Model file for the job. Use its own axes, mm. Round coordinates to 2 decimals unless told otherwise and drop trailing zeros. Loops run counter-clockwise (first coordinate to the right, second up) from the corner with the lowest first, then second, coordinate; pieces in that order, holes last. Notation, with made-up numbers: M 21.5,55.5 L 62.5,55.5 A24 ccw 62.5,71.5 Z; hole C 10.25,8.25 d8. An arc over 180 degrees is marked long. Use a Markdown table: item, result. Add a question column.
Item 1: Pin check, flat tips, straight feed: P1, Ø2, axis at x = 1, y = 12.5, coming from the -Z side; P2, Ø1.8, axis at y = 1.5, z = -2, coming from the -X side; P3, Ø2, axis at x = 0.5, y = 15.5, coming from the +Z side. Stop position of each tip, or through.
Item 2: Saw through at C-C on x = 493. Write the cut outline in (y, z).
Item 3: Saw through at B-B on y = 9. Write the cut outline in (x, z), then the cut area to 3 significant figures.
Item 4: Wall check: L1, parallel to Y at x = 603, z = -174; L2, parallel to Z at x = 384, y = 22.5; L3, parallel to Z at x = 288, y = 27.5. Give the ranges that are in metal, low to high. Write a range as from..to.
Item 5: Saw through at A-A on z = -30. Write the cut outline in (x, y).
Item 6: Two-plate mould, pull along Z, no slides. Class faces 1 (the flat face through (700, 15, -222)), 2 (the flat face through (345, 15, 0)), 3 (the flat face through (345, 2, -222)): +Z half, -Z half, draft (parallel to the pull), parting line (faces both ways), or undercut.
```python
from build123d import *

# Parameters (mm, degrees)
SKETCH2_W                  = 700
SKETCH2_H                  = 450
BOSS_EXTRUDE1_DEPTH        = 30
CONVERT_SOLID1_START       = 3
CONVERT_SOLID1_DEPTH       = 694
CONVERT_SOLID1_2_OUTLINE_W = 24.146446609
CONVERT_SOLID1_2_OUTLINE_H = 2
CONVERT_SOLID1_2_DEPTH     = 2.353553391
CONVERT_SOLID1_START_2     = 697.646446609
CONVERT_SOLID1_3_OUTLINE_W = 24.146446609
CONVERT_SOLID1_3_OUTLINE_H = 2
CONVERT_SOLID1_3_DEPTH     = 2.353553391
CONVERT_SOLID1_4_DEPTH     = 700
CONVERT_SOLID1_5_DEPTH     = 2.353553391
CONVERT_SOLID1_6_DEPTH     = 2.353553391
CONVERT_SOLID1_START_3     = 2.353553391
CONVERT_SOLID1_7_DEPTH     = 1.146446609
CONVERT_SOLID1_START_4     = 696.5
CONVERT_SOLID1_8_DEPTH     = 1.146446609
CONVERT_SOLID1_START_5     = -447.646446609
CONVERT_SOLID1_9_DEPTH     = 445.292893218


with BuildPart() as part:
    # Sketch2 → Boss-Extrude1 (new body)
    with BuildSketch(Plane(origin=(0, 0, 0), x_dir=(1, 0, 0), z_dir=(0, 1, 0))):
        with Locations((350, 225)):
            Rectangle(SKETCH2_W, SKETCH2_H)
    extrude(amount=BOSS_EXTRUDE1_DEPTH)

    # Convert-Solid1: read off the stored shape, not the designer's step
    # Convert-Solid1 outline → Convert-Solid1 (cut)
    with BuildSketch(Plane.YZ.offset(CONVERT_SOLID1_START)):
        with BuildLine():
            Line((3.5, -3.5), (2, -3.5))
            Line((2, -3.5), (2, -446.5))
            Line((2, -446.5), (3.5, -446.5))
            Line((3.5, -446.5), (3.5, -447.646446609))
            Line((3.5, -447.646446609), (27.646446609, -447.646446609))
            Line((27.646446609, -447.646446609), (27.646446609, -3.353553391))
            ThreePointArc((27.646446609, -3.353553391), (27.353553391, -2.646446609), (26.646446609, -2.353553391))
            Line((26.646446609, -2.353553391), (3.5, -2.353553391))
            Line((3.5, -2.353553391), (3.5, -3.5))
        make_face()
    extrude(amount=CONVERT_SOLID1_DEPTH, mode=Mode.SUBTRACT)

    # Convert-Solid1 2 outline → Convert-Solid1 2 (cut)
    with BuildSketch(Plane.YZ):
        with Locations((15.573223305, -449)):
            Rectangle(CONVERT_SOLID1_2_OUTLINE_W, CONVERT_SOLID1_2_OUTLINE_H)
    extrude(amount=CONVERT_SOLID1_2_DEPTH, mode=Mode.SUBTRACT)

    # Convert-Solid1 3 outline → Convert-Solid1 3 (cut)
    with BuildSketch(Plane.YZ.offset(CONVERT_SOLID1_START_2)):
        with Locations((15.573223305, -449)):
            Rectangle(CONVERT_SOLID1_3_OUTLINE_W, CONVERT_SOLID1_3_OUTLINE_H)
    extrude(amount=CONVERT_SOLID1_3_DEPTH, mode=Mode.SUBTRACT)

    # Convert-Solid1 4 outline → Convert-Solid1 4 (cut)
    with BuildSketch(Plane.YZ):
        with BuildLine():
            Line((2, -3), (2, -3.5))
            Line((2, -3.5), (3.5, -3.5))
            Line((3.5, -3.5), (3.5, -2.353553391))
            Line((3.5, -2.353553391), (26.646446609, -2.353553391))
            ThreePointArc((26.646446609, -2.353553391), (27.353553391, -2.646446609), (27.646446609, -3.353553391))
            Line((27.646446609, -3.353553391), (27.646446609, -447.646446609))
            Line((27.646446609, -447.646446609), (3.5, -447.646446609))
            Line((3.5, -447.646446609), (3.5, -446.5))
            Line((3.5, -446.5), (2, -446.5))
            Line((2, -446.5), (2, -447))
            ThreePointArc((2, -447), (2.292893219, -447.707106781), (3, -448))
            Line((3, -448), (27.646446609, -448))
            Line((27.646446609, -448), (27.646446609, -450))
            Line((27.646446609, -450), (30, -450))
            Line((30, -450), (30, -447.646446609))
            Line((30, -447.646446609), (28, -447.646446609))
            Line((28, -447.646446609), (28, -3))
            ThreePointArc((28, -3), (27.707106781, -2.292893219), (27, -2))
            Line((27, -2), (3, -2))
            ThreePointArc((3, -2), (2.292893219, -2.292893219), (2, -3))
        make_face()
        with BuildLine():
            Line((0, 0), (0, -3))
            ThreePointArc((0, -3), (0.878679656, -0.878679656), (3, 0))
            Line((3, 0), (0, 0))
        make_face()
        with BuildLine():
            ThreePointArc((3, -450), (0.878679656, -449.121320344), (0, -447))
            Line((0, -447), (0, -450))
            Line((0, -450), (3, -450))
        make_face()
        with BuildLine():
            Line((30, 0), (27, 0))
            ThreePointArc((27, 0), (29.121320344, -0.878679656), (30, -3))
            Line((30, -3), (30, 0))
        make_face()
    extrude(amount=CONVERT_SOLID1_4_DEPTH, mode=Mode.SUBTRACT)

    # Convert-Solid1 5 outline → Convert-Solid1 5 (cut)
    with BuildSketch(Plane.YZ):
        with BuildLine():
            Line((0, -3), (0, -3.5))
            Line((0, -3.5), (2, -3.5))
            Line((2, -3.5), (2, -3))
            ThreePointArc((2, -3), (2.292893219, -2.292893219), (3, -2))
            Line((3, -2), (27, -2))
            ThreePointArc((27, -2), (27.707106781, -2.292893219), (28, -3))
            Line((28, -3), (28, -447.646446609))
            Line((28, -447.646446609), (30, -447.646446609))
            Line((30, -447.646446609), (30, -3))
            ThreePointArc((30, -3), (29.121320344, -0.878679656), (27, 0))
            Line((27, 0), (3, 0))
            ThreePointArc((3, 0), (0.878679656, -0.878679656), (0, -3))
        make_face()
        with BuildLine():
            Line((2, -446.5), (0, -446.5))
            Line((0, -446.5), (0, -447))
            ThreePointArc((0, -447), (0.878679656, -449.121320344), (3, -450))
            Line((3, -450), (3.5, -450))
            Line((3.5, -450), (3.5, -448))
            Line((3.5, -448), (3, -448))
            ThreePointArc((3, -448), (2.292893219, -447.707106781), (2, -447))
            Line((2, -447), (2, -446.5))
        make_face()
    extrude(amount=CONVERT_SOLID1_5_DEPTH, mode=Mode.SUBTRACT)

    # Convert-Solid1 6 outline → Convert-Solid1 6 (cut)
    with BuildSketch(Plane.YZ.offset(CONVERT_SOLID1_START_2)):
        with BuildLine():
            Line((0, -3), (0, -3.5))
            Line((0, -3.5), (2, -3.5))
            Line((2, -3.5), (2, -3))
            ThreePointArc((2, -3), (2.292893219, -2.292893219), (3, -2))
            Line((3, -2), (27, -2))
            ThreePointArc((27, -2), (27.707106781, -2.292893219), (28, -3))
            Line((28, -3), (28, -447.646446609))
            Line((28, -447.646446609), (30, -447.646446609))
            Line((30, -447.646446609), (30, -3))
            ThreePointArc((30, -3), (29.121320344, -0.878679656), (27, 0))
            Line((27, 0), (3, 0))
            ThreePointArc((3, 0), (0.878679656, -0.878679656), (0, -3))
        make_face()
        with BuildLine():
            Line((2, -446.5), (0, -446.5))
            Line((0, -446.5), (0, -447))
            ThreePointArc((0, -447), (0.878679656, -449.121320344), (3, -450))
            Line((3, -450), (3.5, -450))
            Line((3.5, -450), (3.5, -448))
            Line((3.5, -448), (3, -448))
            ThreePointArc((3, -448), (2.292893219, -447.707106781), (2, -447))
            Line((2, -447), (2, -446.5))
        make_face()
    extrude(amount=CONVERT_SOLID1_6_DEPTH, mode=Mode.SUBTRACT)

    # Convert-Solid1 7 outline → Convert-Solid1 7 (cut)
    with BuildSketch(Plane.YZ.offset(CONVERT_SOLID1_START_3)):
        with BuildLine():
            Line((0, -3), (0, -3.5))
            Line((0, -3.5), (2, -3.5))
            Line((2, -3.5), (2, -3))
            ThreePointArc((2, -3), (2.292893219, -2.292893219), (3, -2))
            Line((3, -2), (3.5, -2))
            Line((3.5, -2), (3.5, 0))
            Line((3.5, 0), (3, 0))
            ThreePointArc((3, 0), (0.878679656, -0.878679656), (0, -3))
        make_face()
        with BuildLine():
            Line((2, -446.5), (0, -446.5))
            Line((0, -446.5), (0, -447))
            ThreePointArc((0, -447), (0.878679656, -449.121320344), (3, -450))
            Line((3, -450), (3.5, -450))
            Line((3.5, -450), (3.5, -448))
            Line((3.5, -448), (3, -448))
            ThreePointArc((3, -448), (2.292893219, -447.707106781), (2, -447))
            Line((2, -447), (2, -446.5))
        make_face()
    extrude(amount=CONVERT_SOLID1_7_DEPTH, mode=Mode.SUBTRACT)

    # Convert-Solid1 8 outline → Convert-Solid1 8 (cut)
    with BuildSketch(Plane.YZ.offset(CONVERT_SOLID1_START_4)):
        with BuildLine():
            Line((0, -3), (0, -3.5))
            Line((0, -3.5), (2, -3.5))
            Line((2, -3.5), (2, -3))
            ThreePointArc((2, -3), (2.292893219, -2.292893219), (3, -2))
            Line((3, -2), (3.5, -2))
            Line((3.5, -2), (3.5, 0))
            Line((3.5, 0), (3, 0))
            ThreePointArc((3, 0), (0.878679656, -0.878679656), (0, -3))
        make_face()
        with BuildLine():
            Line((2, -446.5), (0, -446.5))
            Line((0, -446.5), (0, -447))
            ThreePointArc((0, -447), (0.878679656, -449.121320344), (3, -450))
            Line((3, -450), (3.5, -450))
            Line((3.5, -450), (3.5, -448))
            Line((3.5, -448), (3, -448))
            ThreePointArc((3, -448), (2.292893219, -447.707106781), (2, -447))
            Line((2, -447), (2, -446.5))
        make_face()
    extrude(amount=CONVERT_SOLID1_8_DEPTH, mode=Mode.SUBTRACT)

    # Convert-Solid1 9 outline → Convert-Solid1 9 (cut)
    with BuildSketch(Plane.XY.offset(CONVERT_SOLID1_START_5)):
        with BuildLine():
            Line((0, 0), (3, 0))
            ThreePointArc((3, 0), (0.878679656, 0.878679656), (0, 3))
            Line((0, 3), (0, 0))
        make_face()
        with BuildLine():
            ThreePointArc((700, 3), (699.121320344, 0.878679656), (697, 0))
            Line((697, 0), (700, 0))
            Line((700, 0), (700, 3))
        make_face()
        with BuildLine():
            Line((697, 27.646446609), (697, 2))
            ThreePointArc((697, 2), (697.707106781, 2.292893219), (698, 3))
            Line((698, 3), (698, 27.646446609))
            Line((698, 27.646446609), (697, 27.646446609))
        make_face()
        with BuildLine():
            Line((3, 2), (3, 27.646446609))
            Line((3, 27.646446609), (2, 27.646446609))
            Line((2, 27.646446609), (2, 3))
            ThreePointArc((2, 3), (2.292893219, 2.292893219), (3, 2))
        make_face()
    extrude(amount=CONVERT_SOLID1_9_DEPTH, mode=Mode.SUBTRACT)


solid = part.part
```
Entries:
| question | item | result |
|---|---|---|
| 1 | P1 | z = -447.65 |
| 1 | P2 | x = 3.5 |
| 1 | P3 | z = -2.35 |
| 2 | outline | M 0,-447 A3 ccw 3,-450 L 27.65,-450 L 27.65,-448 L 3,-448 A1 cw 2,-447 L 2,-3 A1 cw 3,-2 L 27,-2 A1 cw 28,-3 L 28,-447.65 L 30,-447.65 L 30,-3 A3 ccw 27,0 L 3,0 A3 ccw 0,-3 Z |
| 3 | outline | M 0,-447.65 L 2,-447.65 L 2,-2.35 L 0,-2.35 Z; M 2.35,-450 L 697.65,-450 L 697.65,-448 L 2.35,-448 Z; M 2.35,-2 L 697.65,-2 L 697.65,0 L 2.35,0 Z; M 698,-447.65 L 700,-447.65 L 700,-2.35 L 698,-2.35 Z |
| 3 | area | 4,560 mm2 |
| 4 | L1 | 0..2, 28..30 |
| 4 | L2 | -450..-448, -2..0 |
| 4 | L3 | -450..-448, -2.13..-0.04 |
| 5 | outline | M 0,3 A3 ccw 3,0 L 697,0 A3 ccw 700,3 L 700,27.65 L 698,27.65 L 698,3 A1 cw 697,2 L 3,2 A1 cw 2,3 L 2,27.65 L 0,27.65 Z; M 2.35,28 L 697.65,28 L 697.65,30 L 2.35,30 Z |
| 6 | face 1 | draft |
| 6 | face 2 | +Z half |
| 6 | face 3 | undercut |
